The model under review builds one solid part; all positions refer to its coordinate system, in mm. Face numbers are marked on the shaded views. A direction names the side the tool comes from. Round coordinates to 2 decimals unless told otherwise and drop trailing zeros. Write each loop counter-clockwise with the first axis right and the second up, starting at its lowest first coordinate (ties: lowest second). Pieces come first, ordered by that corner, then holes. Notation, with made-up numbers: (-26.75, 76.25) -> (21.25, 76.25) arc R12 ccw to (21.25, 82.25) -> close; hole circle Ø6 at (-38, 42). An arc over 180 degrees is marked (long way). Return JSON: item names as keys, results as strings. Group by question number.
1. For line 1 along Y through (x, z) = (36.95, 2.95) (3 decimals); line 2 along Z through (x, y) = (10, -37); line 3 along X through (y, z) = (-39, -37.5) (1 decimal), list the stretches that pass through material, from the lowest coordinate up. Write a range as from..to.
2. Mouldability with a two-part tool opening along Z and no side actions: class the marked faces 1, 2 and 3 as pulls with the +Z half, pulls with the -Z half, needs draft (parallel to the pull), parting line crosses it, or undercut.
3. Take a section at B-B, the plane y = -55.5. Write out the cut boundary in (x, z) (1 decimal), then the cut area to 3 significant figures.
4. Take a section at C-C, the plane y = 0. Give the number of separate pieces and of enclosed holes in the cut face, then the cut area to 3 significant figures.
5. Clearance check with flat-ended pins moving along their axes: P1, Ø5, axis at x = -20.5, z = 2, coming from the -Y side (3 decimals); P2, Ø2, axis at y = 7, z = -26, coming from the -X side; P3, Ø8, axis at y = -31.5, z = -33, coming from the +X side (3 decimals); P4, Ø17.5, axis at x = -15.12, y = -50.29, coming from the +Z side. State where each tip first meets the part, or that it passes through.
6. Tool access review of the marked faces 4, 5, 6 and 7: name each direction out of +Z, -Z, +X, -X, +Y, -Y from which nothing blocks a thin tool from reaching the whole face with its end or side.
7. Take a section at D-D, the plane z = -38.5. Write out the cut boundary in (x, y) (1 decimal).
8. Take a section at A-A, the plane x = 36.95. Write out the cut boundary in (y, z) (1 decimal), then the cut area to 3 significant figures.
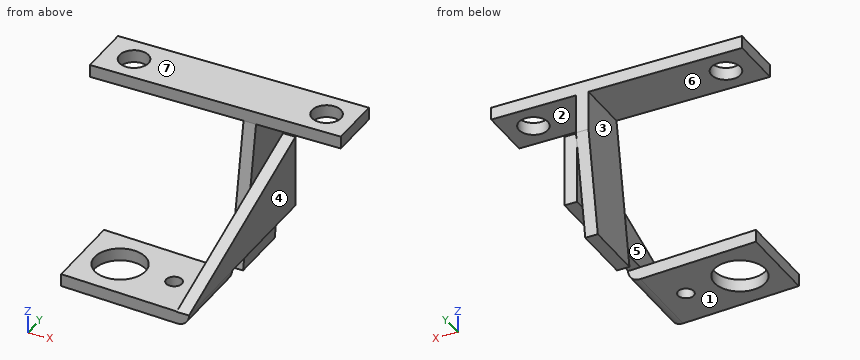
Autodesk Fusion 360 part; units mm, degrees
sketch "Sketch4" plane through (0, 0, 0) normal (0, 0, 1) x (1, 0, 0)
  line L0 (-47.7, 10.125) -> (47.7, 10.125)
  line L1 (47.7, 10.125) -> (47.7, -10.125)
  line L2 (47.7, -10.125) -> (-47.7, -10.125)
  line L3 (-47.7, -10.125) -> (-47.7, 10.125)
  line L4 (-47.7, 0) -> (47.7, 0) construction
  circle A0 centre (36.95, 0) radius 5.5
  line L5 (0.3455, 47) -> (0.3455, -29) construction
  circle A1 centre (-36.2591, 0) radius 5.5
  line L6 (42.45, 3.7083) -> (42.45, -3.7083) construction
  point P0 (47.7, 0)
  point P1 (-47.7, 0)
  point P2 (42.45, 0)
  dimension "d16" = 95.4
  dimension "d17" = 20.25
  dimension "d18" = 11
  dimension "d20" = 5.25
extrude "Extrude2" add sketch "Sketch4" along normal blind 4.7625
sketch "Sketch5" plane through (0, 0, 0) normal (0, 0, -1) x (1, 0, 0)
  circle A0 centre (36.95, 0) radius 5.5
  circle A1 centre (-36.2591, 0) radius 5.5
  line L0 (47.7, 10.125) -> (-47.7, 10.125)
  line L1 (-47.7, 10.125) -> (-47.7, -10.125)
  line L2 (-47.7, -10.125) -> (47.7, -10.125)
  line L3 (47.7, -10.125) -> (47.7, 10.125)
  line L4 (10.7, 15.5999) -> (15.4625, 15.5999)
  line L5 (15.4625, 15.5999) -> (15.4625, -14.8215)
  line L6 (10.7, -14.8215) -> (10.7, 15.5999)
  line L7 (10.7, -14.8215) -> (15.4625, -14.8215)
  dimension "d24" = 37
  dimension "d25" = 4.7625
extrude "Extrude3" add sketch "Sketch5" along normal blind 53.2375 contours L0 L2 L5 L6 | L0 L4 L5 L6 | L2 L5 L6 L7
sketch "Sketch6" plane through (15.4625, 0, 0) normal (1, 0, 0) x (0, 1, 0)
  line L0 (-10.125, 0) -> (-15.5999, 0)
  line L1 (-15.5999, 0) -> (-15.5999, -53.2375)
  line L2 (-15.5999, -53.2375) -> (14.8215, -53.2375)
  line L3 (14.8215, -53.2375) -> (14.8215, 0)
  line L4 (14.8215, 0) -> (10.125, 0)
  line L5 (10.125, 0) -> (-10.125, 0)
  line L6 (-10.125, 0) -> (10.125, 0)
  line L7 (10.125, 0) -> (10.125, -15)
  line L8 (-10.125, 0) -> (-19.5122, -53.2375)
  line L9 (10.125, -15) -> (3.3827, -53.2375)
  line L10 (-19.5122, -53.2375) -> (3.3827, -53.2375)
  point P0 (10.125, 0)
  dimension "d30" = 100
extrude "Extrude4" cut sketch "Sketch6" against normal up to surface (4.7625 mm away) contours L0 L1 L8 | L2 L3 L4 L7 L9
extrude "Extrude5" add sketch "Sketch6" against normal up to surface (4.7625 mm away) contours L1 L8 L10
sketch "Sketch7" plane through (15.4625, 0, 0) normal (1, 0, 0) x (0, 1, 0)
  line L0 (3.3827, -53.2375) -> (10.125, -15)
  line L1 (10.125, -15) -> (10.125, 0)
  line L2 (10.125, 0) -> (-10.125, 0)
  line L3 (-10.125, 0) -> (-19.5122, -53.2375)
  line L4 (-19.5122, -53.2375) -> (3.3827, -53.2375)
  line L5 (-67.6425, -42.2375) -> (9.3575, -14.7375)
  line L6 (9.3575, -14.7375) -> (9.3575, -42.2375)
  line L7 (9.3575, -42.2375) -> (-67.6425, -42.2375)
  line L8 (-10.125, 4.7625) -> (10.125, 4.7625)
  dimension "d35" = 77
  dimension "d36" = 27.5
  dimension "d37" = 47
extrude "Extrude6" add sketch "Sketch7" along normal blind 4.7625 contours L0 L3 L5 L6 L7 | L0 L6 L7 | L3 L5 L7
sketch "Sketch8" plane through (0, 0, -42.2375) normal (0, 0, -1) x (1, 0, 0)
  line L0 (15.4625, -5.3223) -> (15.4625, -9.3575)
  line L1 (15.4625, -9.3575) -> (20.225, -9.3575)
  line L2 (20.225, -9.3575) -> (20.225, 67.6425)
  line L3 (20.225, 67.6425) -> (15.4625, 67.6425)
  line L4 (15.4625, 67.6425) -> (15.4625, 17.5726)
  line L5 (15.4625, 17.5726) -> (15.4625, -5.3223)
  line L6 (20.225, 67.6425) -> (-29.775, 65.0221)
  line L7 (-29.775, 65.0221) -> (-29.775, 34.0221)
  line L8 (-29.775, 34.0221) -> (20.225, 36.6425)
  line L9 (20.225, 36.6425) -> (20.225, 67.6425)
  circle A0 centre (-15.125, 50.2899) radius 9.65
  line L10 (-15.125, 40.6399) -> (-15.125, 59.9399) construction
  line L11 (-5.475, 50.2899) -> (-24.775, 50.2899) construction
  line L12 (-24.775, 58.5104) -> (-24.775, 42.0694) construction
  line L13 (-15.1316, 59.9399) -> (-15.1184, 59.9399) construction
  line L14 (-15.1316, 40.6399) -> (-15.1184, 40.6399) construction
  line L15 (-15.9351, 65.7475) -> (-14.3149, 34.8324) construction
  line L16 (15.4625, 51.8929) -> (-29.775, 49.5221) construction
  circle A1 centre (5.996, 51.3968) radius 3
  line L17 (-5.6407, 53.7042) -> (-5.3358, 47.8857) construction
  line L18 (2.8046, 54.9702) -> (3.1956, 47.5094) construction
  point P0 (-15.125, 50.2899)
  point P1 (-5.4882, 50.795)
  point P2 (3.0001, 51.2398)
  dimension "d40" = 3
  dimension "d41" = 50
  dimension "d42" = 31
  dimension "d44" = 19.3
  dimension "d45" = 5
  dimension "d47" = 30.9575
  dimension "d49" = 6
  dimension "d50" = 8.5
extrude "Extrude7" add sketch "Sketch8" along normal blind 4.7625 contours L4 L6 L7 L8 | L2 L4 L6 L8 L9
fillet "Fillet1" radius 4.7625 1 edges at (20.225, -52.1425, -47)
equation "d21 = ( 3 / 16 ) * 1 in"
equation "d25 = ( 3 / 16 ) * 1 in"
equation "d26 = 58 mm - ( ( 3 / 16 ) * 1 in )"
equation "d30 = 90 deg + 10 deg"
equation "d38 = ( 3 / 16 ) * 1 in"
equation "d51 = ( 3 / 16 ) * 1 in"
equation "d54 = ( 3 / 16 ) * 1 in"
Output:
{
 "1": {"line 1": "y = -10.125..-5.5, 5.5..10.125", "line 2": "z = -47..-42.24", "line 3": "x = 15.5..20.2"},
 "2": {"face 1": "pulls with the -Z half", "face 2": "undercut", "face 3": "needs draft"},
 "3": {"outline": "(-29.8, -47) -> (-23.2, -47) -> (-23.2, -42.2) -> (-29.8, -42.2) -> close; (-7, -47) -> (15.5, -47) arc R4.8 ccw to (20.2, -42.2) -> (20.2, -37.9) -> (15.5, -37.9) -> (15.5, -42.2) -> (-7, -42.2) -> close", "area": "177 mm^2"},
 "4": {"separate pieces": "3", "enclosed holes": "0", "area": "718 mm^2"},
 "5": {"P1": "stops at y = -10.125", "P2": "stops at x = 10.7", "P3": "stops at x = 20.225", "P4": "passes through"},
 "6": {"face 4": "-Z, +X, +Y, -Y", "face 5": "+Z, -X, -Y", "face 6": "-Z, -X, +Y, -Y", "face 7": "+Z, +X, -X, +Y, -Y"},
 "7": {"outline": "(10.7, -16.9) -> (15.5, -16.9) -> (15.5, -57.2) -> (20.2, -57.2) -> (20.2, 9.4) -> (15.5, 9.4) -> (15.5, 6) -> (10.7, 6) -> close"},
 "8": {"outline": "(-10.1, 0) -> (-5.5, 0) -> (-5.5, 4.8) -> (-10.1, 4.8) -> close; (5.5, 0) -> (10.1, 0) -> (10.1, 4.8) -> (5.5, 4.8) -> close", "area": "44.1 mm^2"}
}
